Geometry: final body of the model. Coordinates: model frame, mm. Face numbers are marked on the shaded views. A direction names the side the tool comes from. Coordinates: 2 decimals unless noted, no trailing zeros. Write each loop counter-clockwise with the first axis right and the second up, starting at its lowest first coordinate (ties: lowest second). Pieces come first, ordered by that corner, then holes.
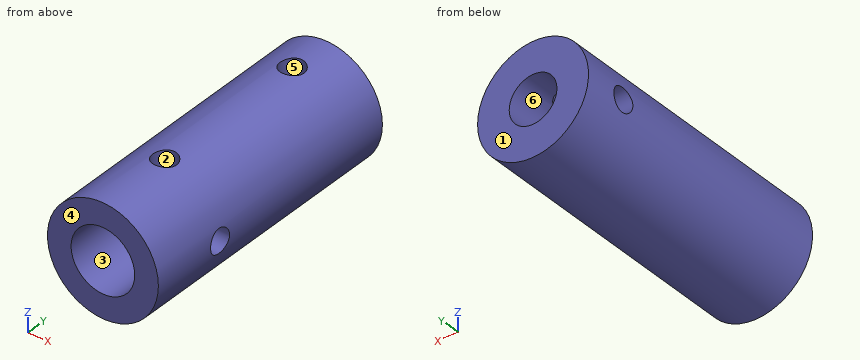
Solid Edge part; units mm, degrees
sketch "Sketch1" plane through (0, 0, 0) normal (0, -1, 0) x (1, 0, 0)
  circle A0 centre (0, 0) radius 6.975
extrude "Protrusion1" add sketch "Sketch1" along normal blind 35.39
sketch "Sketch2" plane through (0, -35.39, 0) normal (0, -1, 0) x (1, 0, 0)
  circle A0 centre (0, 0) radius 3
extrude "Cutout1" cut sketch "Sketch2" against normal through all
sketch "Sketch3" plane through (0, -35.39, 0) normal (0, -1, 0) x (1, 0, 0)
  circle A0 centre (0, 0) radius 4
extrude "ExtrudedCutout_2" cut sketch "Sketch3" against normal blind 16.35
sketch "Sketch4" plane through (0, 0, 0) normal (0, 0, 1) x (1, 0, 0)
  circle A0 centre (0, -25.64) radius 1.5
  circle A1 centre (0, -5.51) radius 1.5
extrude "ExtrudedCutout_3" cut sketch "Sketch4" along normal blind 12.2726
sketch "Sketch5" plane through (0, 0, 0) normal (1, 0, 0) x (0, 1, 0)
  circle A0 centre (-25.64, 0) radius 1.5
extrude "ExtrudedCutout_4" cut sketch "Sketch5" along normal blind 9.4946
sketch "Sketch6" plane through (0, 0, 0) normal (1, 0, 0) x (0, 1, 0)
  circle A0 centre (-5.51, 0) radius 1.5
extrude "ExtrudedCutout_5" cut sketch "Sketch6" against normal blind 15.7832
properties material "Aluminum, 5050"
Item 1: Section B-B, the plane z = 0. Output: boundary loops of the cut face in (x, y) (3 decimals), plus the area to 3 significant figures.
Derived:
outline: (-6.975, -35.39) - (-4, -35.39) - (-4, -19.04) - (-3, -19.04) - (-3, -7.01) - (-6.975, -7.01) - close; (-6.975, -4.01) - (-3, -4.01) - (-3, 0) - (-6.975, 0) - close; (3, -19.04) - (4, -19.04) - (4, -24.14) - (6.975, -24.14) - (6.975, 0) - (3, 0) - close; (4, -35.39) - (6.975, -35.39) - (6.975, -27.14) - (4, -27.14) - close
area: 228 mm2
Item 2: Section A-A, the plane x = 0. Output: boundary loops of the cut face in (y, z) (3 decimals).
Derived:
outline: (-35.39, -6.975) - (0, -6.975) - (0, -3) - (-19.04, -3) - (-19.04, -4) - (-35.39, -4) - close; (-35.39, 4) - (-27.14, 4) - (-27.14, 6.975) - (-35.39, 6.975) - close; (-24.14, 4) - (-19.04, 4) - (-19.04, 3) - (-7.01, 3) - (-7.01, 6.975) - (-24.14, 6.975) - close; (-4.01, 3) - (0, 3) - (0, 6.975) - (-4.01, 6.975) - close
Item 3: Section C-C, the plane y = -5.51. Output: boundary loops of the cut face in (x, z) (3 decimals).
Derived:
outline: (-6.812, -1.5) arc R6.975 ccw (long way) to (1.5, 6.812) - (1.5, 2.598) arc R3 cw (long way) to (-2.598, -1.5) - close; (-6.812, 1.5) - (-2.598, 1.5) arc R3 cw to (-1.5, 2.598) - (-1.5, 6.812) arc R6.975 ccw to start
Item 4: Material intervals for probe 1 along Y at (x, z) = (0, 4.4); probe 2 along Z at (x, y) = (0, -12.5) (3 decimals); probe 3 along Y at (x, z) = (0, 3.9), sorted ascending.
Derived:
probe 1: y = -35.39 to -27.14, -24.14 to -7.01, -4.01 to 0
probe 2: z = -6.975 to -3, 3 to 6.975
probe 3: y = -19.04 to -7.01, -4.01 to 0
Item 5: Pin query (flat end, axial travel): pin 1 (1.5 mm diameter, centred on y = -9, z = -1, fed in from +X); pin 2 (1 mm diameter, centred on y = -7.5, z = -2, fed in from -X); pin 3 (3 mm diameter, centred on x = -5, y = -24.5, fed in from -Z). Return the tip coordinate at first contact, or that it passes through.
Derived:
pin 1: stops at x = 6.97
pin 2: stops at x = -6.81
pin 3: stops at z = -6.03
Item 6: Pull-direction query (Y, two-part tool) for the marked faces 1, 2, 3 and 4; classes: released by +Y, released by -Y, zero draft, split by the parting line, or undercut.
Derived:
face 1: released by +Y
face 2: undercut
face 3: zero draft
face 4: released by -Y
Item 7: Section D-D, the plane z = -2. Output: boundary loops of the cut face in (x, y), plus the area to 3 significant figures.
Derived:
outline: (-6.68, -35.39) - (-3.46, -35.39) - (-3.46, -19.04) - (-2.24, -19.04) - (-2.24, 0) - (-6.68, 0) - close; (2.24, -19.04) - (3.46, -19.04) - (3.46, -35.39) - (6.68, -35.39) - (6.68, 0) - (2.24, 0) - close
area: 275 mm2
Item 8: Set-up query: the marked faces 5 and 6. Return all of +Z, -Z, +X, -X, +Y, -Y with unobstructed straight access to the full face (end or side cutting, diameter ignored); none if empty.
Derived:
face 5: +Z
face 6: +Y, -Y
